Work out the finished part from the listing and answer in its coordinate system (mm). A direction names the side the tool comes from. Round coordinates to 2 decimals unless told otherwise and drop trailing zeros. Write each loop counter-clockwise with the first axis right and the second up, starting at its lowest first coordinate (ties: lowest second). Pieces come first, ordered by that corner, then holes. Notation, with made-up numbers: (-2, 71.5) -> (34, 71.5) arc R13 cw to (34, 80.5) -> close; hole circle Ø2 at (0, 52.5). An arc over 180 degrees is marked (long way). Answer as a JSON object with one key per item and string values. Group by question number.
Autodesk Inventor part; units mm, degrees
ref_plane "YZ Plane" through (0, 0, 0) normal (1, 0, 0) x (0, 1, 0)
ref_plane "XZ Plane" through (0, 0, 0) normal (0, 1, 0) x (-1, 0, 0)
ref_plane "XY Plane" through (0, 0, 0) normal (0, 0, 1) x (1, 0, 0)
sketch "_____1" plane through (0, 0, 0) normal (0, 0, 1) x (1, 0, 0)
  line L0 (50, 0) -> (-50, 0)
  line L1 (-1.25, 0) -> (-1.25, 2.94)
  line L2 (-1.25, 2.94) -> (-1.1, 2.94)
  line L3 (-1.1, 2.94) -> (-1.1, 3.46)
  line L4 (-1.1, 3.46) -> (-1.25, 3.46)
  line L5 (-1.25, 3.46) -> (-1.25, 3.9)
  arc A0 (-1.15, 4) -> (-1.25, 3.9) centre (-1.15, 3.9) ccw
  line L6 (-1.15, 4) -> (0.65, 4)
  line L7 (0.65, 4) -> (0.65, 4.6)
  line L8 (0.65, 4.6) -> (1.25, 4.6)
  line L9 (1.25, 4.6) -> (1.25, 3.46)
  line L10 (1.25, 3.46) -> (1.1, 3.46)
  line L11 (1.1, 3.46) -> (1.1, 2.94)
  line L12 (1.1, 2.94) -> (1.25, 2.94)
  line L13 (1.25, 2.94) -> (1.25, 0)
  line L14 (1.25, 0) -> (-1.25, 0)
revolve "Revolution1" add sketch "_____1" angle 360 about axis through (50, 0, 0) along (1, 0, 0)
sketch "_____2" plane through (0, 0, 0) normal (0, 0, 1) x (1, 0, 0)
  line L0 (50, 0) -> (-50, 0)
  line L1 (-1.25, 0) -> (-1.25, 2.6)
  arc A0 (-1.25, 2.6) -> (-1.15, 2.5) centre (-1.15, 2.6) ccw
  line L2 (-1.15, 2.5) -> (1.15, 2.5)
  arc A1 (1.15, 2.5) -> (1.25, 2.6) centre (1.15, 2.6) ccw
  line L3 (1.25, 2.6) -> (1.25, 0)
  line L4 (1.25, 0) -> (-1.25, 0)
revolve "Revolution2" cut sketch "_____2" angle 360 about axis through (50, 0, 0) along (1, 0, 0)
properties part number "C-FL675ZZ"
1) For a pull along Y with two mould halves and no side action, classify faces 1 (the face through (0.95, -3.65, -2.8)), 2 (the face through (0.02, -0.54, -2.44)), 3 (the face through (0.65, -1.7, 3.8)) as released by +Y, released by -Y, zero draft, split by the parting line, or undercut.
2) Straight lines are drawn through the part: L1, parallel to Z at x = 0.7, y = 0; L2, parallel to Z at x = 1.2, y = 0; L3, parallel to X at y = -3.75, z = -1.75. For each, find the intervals that lie inside material, in ascending order.
3) A tool of negligible diameter and unlimited length cuts with its end or side. For faces 4 (the face through (1.1, -1, -3)), 5 (the face through (-0.237, -0.867, -3.905)), from which of +Z, -Z, +X, -X, +Y, -Y can it reach the whole face along a straight path? Write none if from no direction.
4) A cutting plane is placed at C-C on x = 0.05. Determine the outline of the cut face in (y, z).
5) A cutting plane is placed at D-D on y = 4.25. Determine the outline of the cut face in (x, z).
Established:
{
 "1": {"face 1": "split by the parting line", "face 2": "undercut", "face 3": "zero draft"},
 "2": {"L1": "z = -4.6 to -2.5, 2.5 to 4.6", "L2": "z = -4.6 to -3.46, -2.94 to -2.51, 2.51 to 2.94, 3.46 to 4.6", "L3": "x = 0.65 to 1.25"},
 "3": {"face 4": "+X", "face 5": "-X"},
 "4": {"outline": "circle Ø8 at (0, 0); hole circle Ø5 at (0, 0)"},
 "5": {"outline": "(0.65, -1.76) -> (1.25, -1.76) -> (1.25, 1.76) -> (0.65, 1.76) -> close"}
}
